Check sheet for the modelled part. Datum: model origin and axes. Units: mm. A direction names the side the tool comes from. Round coordinates to 2 decimals unless told otherwise and drop trailing zeros. Write each loop counter-clockwise with the first axis right and the second up, starting at its lowest first coordinate (ties: lowest second). Pieces come first, ordered by that corner, then holes. Notation, with made-up numbers: M 37.5,-27.5 L 50.5,-27.5 A25 ccw 50.5,3.5 Z; hole C -5.75,-40 d5. An arc over 180 degrees is marked long. Put each result on its own line as item: value.
```python
from build123d import *

# Parameters (mm, degrees)
F0_W     = 127
F0_H     = 12.6365
F3_DEPTH = 25.4
F4_R     = 3.175
F5_DEPTH = 12.7


with BuildPart() as f1:
    # F0 (on Front) → F1 (revolve)
    with BuildSketch(Plane.XZ):
        with Locations((69.85, 6.31825)):
            Rectangle(F0_W, F0_H)
    revolve(axis=Axis((-3.592643, 0, 0), (1, 0, 0)))

    # F2 (on face) → F3 (cut)
    with BuildSketch(Plane.YZ.offset(133.35)):
        with BuildLine():
            ThreePointArc((6.35, -10.998523), (12.7, 0), (6.35, 10.998523))
            Line((6.35, 10.998523), (6.35, -10.998523))
        make_face()
        with BuildLine():
            Line((-6.35, -10.998523), (-6.35, 10.998523))
            ThreePointArc((-6.35, 10.998523), (-12.7, 0), (-6.35, -10.998523))
        make_face()
    extrude(amount=-F3_DEPTH, mode=Mode.SUBTRACT)

    # F4 (on Front) → F5 (cut, symmetric)
    with BuildSketch(Plane.XZ):
        with Locations((127, 0)):
            Circle(F4_R)
    extrude(amount=F5_DEPTH, both=True, mode=Mode.SUBTRACT)

    # F6 (on face) → F7 (revolve, cut)
    with BuildSketch(Plane(origin=(6.35, 0, 0), x_dir=(0, -1, 0), z_dir=(-1, 0, 0))):
        with BuildLine():
            Line((0, 12.7), (0, -12.7))
            ThreePointArc((0, -12.7), (12.7, 0), (0, 12.7))
        make_face()
    revolve(axis=Axis((6.35, 0, -4.069372), (0, 0, -1)), mode=Mode.SUBTRACT)


solid = f1.part
```
1. Cross-section at D-D (x = 105.5). Enter the section's corners in (y, z), then the cut area to 3 significant figures.
Computed values:
outline: C 0,0 d25.27
area: 502 mm2
2. Depth check by flat-ended pin: pin 1 Ø10 at (x, z) = (127, 0) entering from +Y; pin 2 Ø4 at (x, z) = (89, -4.5) entering from -Y; pin 3 Ø4 at (x, z) = (62, 6) entering from -Y. Enter the tip coordinate at first touch or a pass-through.
Computed values:
pin 1: stops at y = 6.35
pin 2: stops at y = -12.39
pin 3: stops at y = -11.99
3. Scan lines: probe 1 along Z at (x, y) = (127, -1.5) (3 decimals); probe 2 along Y at (x, z) = (121, -8.5); probe 3 along Z at (x, y) = (60.5, -7.5). Record each from-to range of solid material in increasing order.
Computed values:
probe 1: z = -12.547 to -3.175, 3.175 to 12.547
probe 2: y = -6.35 to 6.35
probe 3: z = -10.17 to 10.17
4. Release check for a two-part mould opening along Z. For faces 1 (the cylindrical face through (57.394, 4.84, 11.673)), 2 (the cylindrical face through (129.93, -0.09, -1.22)), 3 (the flat face through (121, 6.35, 0)) record: +Z half, -Z half, draft (parallel to the pull), parting line (faces both ways), or undercut.
Computed values:
face 1: parting line
face 2: undercut
face 3: draft
5. Cross-section at C-C (z = -6). Enter the section's corners in (x, y), then the cut area to 3 significant figures.
Computed values:
outline: M 7.62,-11.12 L 107.95,-11.12 L 107.95,-6.35 L 133.35,-6.35 L 133.35,6.35 L 107.95,6.35 L 107.95,11.12 L 7.62,11.12 A11.19 cw Z
area: 2,390 mm2
6. Access from +Z, -Z, +X, -X, +Y, -Y to the whole of each face (thin tool, end or side, straight path). Record for faces 4 (the flat face through (133.35, 0, 0)), 5 (the flat face through (107.95, 9, 0)), 6 (the flat face through (121, -6.35, 0)).
Computed values:
face 4: +Z, -Z, +X, +Y, -Y
face 5: +Z, -Z, +X, +Y
face 6: +Z, -Z, +X, -Y
